Verification items for this drawing (mm, ordinates from the low corner). A direction names the side the tool comes from. Coordinates: 2 decimals unless noted, no trailing zeros. Order: outer loops, then holes, each group sorted by start corner. A loop starts at its lowest first (then second) coordinate and runs counter-clockwise, first axis right, second up. Notation, with made-up numbers: M 59.25,-17.5 L 104.25,-17.5 A28 cw 104.25,1.5 Z; hole C 76.5,9.5 d11. An arc over 180 degrees is marked long. One line per item, written item: value. Start each with the question number.
1) Sectioned sample at A-A, the plane x = 29.56. Enter the section's corners in (y, z), then the cut area to 3 significant figures.
2) Draft check along X on the marked faces 3 and 4. Enter one of: pulls with the +X half, pulls with the -X half, needs draft (parallel to the pull), parting line crosses it, or undercut.
3) Go/stop test with flat-tipped pins: P1, Ø2, axis at x = 40, y = 13, coming from the +Z side; P2, Ø0.9, axis at y = 10.5, z = 3, coming from the +X side; P3, Ø5, axis at x = 29.56, y = 12, coming from the -Z side; P4, Ø6.5, axis at x = 29.56, y = 29.56, coming from the -Z side. Record where each tip stops, or that it passes through.
4) Sectioned sample at B-B, the plane y = 29.56. Enter the section's corners in (x, z).
5) Access from +Z, -Z, +X, -X, +Y, -Y to the whole of each face (thin tool, end or side, straight path). Record for the marked faces 1 and 2.
6) Sectioned sample at D-D, the plane y = 21. Enter the section's corners in (x, z).
7) Sectioned sample at C-C, the plane z = 0.5. Enter the section's corners in (x, y), then the cut area to 3 significant figures.
8) Thickness scan on L1, parallel to Y at x = 12, z = 3.65; L2, parallel to X at y = 29.56, z = 3.3; L3, parallel to X at y = 31, z = 3.2. Record the ranges inside material, lowest first. Write a range as from..to.
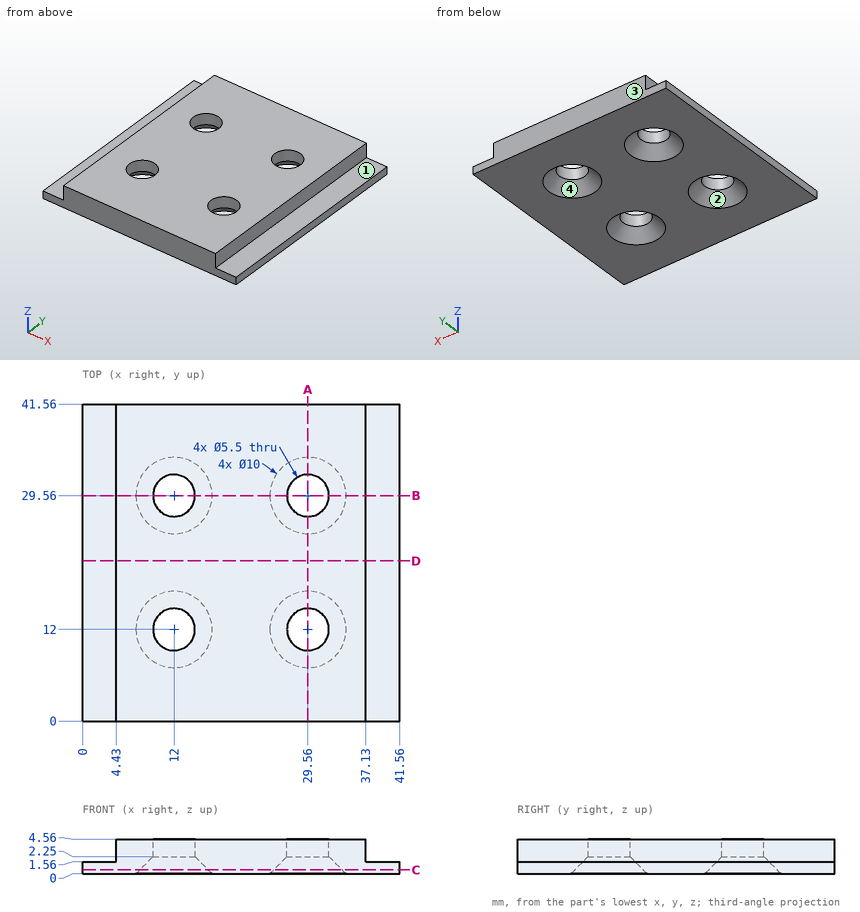
Final values:
1. outline: M 0,0 L 7,0 L 9.25,2.25 L 9.25,4.56 L 0,4.56 Z; M 14.75,2.25 L 17,0 L 24.56,0 L 26.81,2.25 L 26.81,4.56 L 14.75,4.56 Z; M 32.31,2.25 L 34.56,0 L 41.56,0 L 41.56,4.56 L 32.31,4.56 Z
1. area: 129 mm^2
2. face 3: needs draft
2. face 4: undercut
3. P1: stops at z = 1.56
3. P2: stops at x = 37.13
3. P3: passes through
3. P4: stops at z = 1.75
4. outline: M 0,0 L 7,0 L 9.25,2.25 L 9.25,4.56 L 4.43,4.56 L 4.43,1.56 L 0,1.56 Z; M 14.75,2.25 L 17,0 L 24.56,0 L 26.81,2.25 L 26.81,4.56 L 14.75,4.56 Z; M 32.31,2.25 L 34.56,0 L 41.56,0 L 41.56,1.56 L 37.13,1.56 L 37.13,4.56 L 32.31,4.56 Z
5. face 1: +Z, +X, +Y, -Y
5. face 2: -Z
6. outline: M 0,0 L 41.56,0 L 41.56,1.56 L 37.13,1.56 L 37.13,4.56 L 4.43,4.56 L 4.43,1.56 L 0,1.56 Z
7. outline: M 0,0 L 41.56,0 L 41.56,41.56 L 0,41.56 Z; hole C 12,12 d9; hole C 12,29.56 d9; hole C 29.56,12 d9; hole C 29.56,29.56 d9
7. area: 1,470 mm^2
8. L1: y = 0..9.25, 14.75..26.81, 32.31..41.56
8. L2: x = 4.43..9.25, 14.75..26.81, 32.31..37.13
8. L3: x = 4.43..9.66, 14.34..27.22, 31.9..37.13
